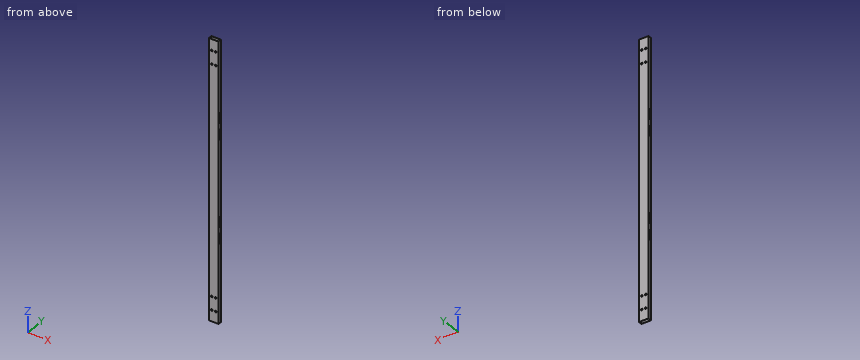
from build123d import *

# Parameters (mm, degrees)
SKETCH_1_W          = 40
SKETCH_1_H          = 15
SKETCH_1_W_2        = 38
SKETCH_1_H_2        = 13
EXTRUDE_1_DEPTH     = 1150
SKETCH_2_R          = 3.575
CUT_EXTRUDE_1_DEPTH = 1151.793204707
SKETCH_3_R          = 2.1
CUT_EXTRUDE_2_DEPTH = 1151.793204707


with BuildPart() as part:
    # 草图1 → 凸台-拉伸1 (new body)
    with BuildSketch(Plane.XY):
        with Locations((20, 7.5)):
            Rectangle(SKETCH_1_W, SKETCH_1_H)
        with Locations((20, 7.5)):
            Rectangle(SKETCH_1_W_2, SKETCH_1_H_2, mode=Mode.SUBTRACT)
    extrude(amount=EXTRUDE_1_DEPTH)

    # 草图2 → 切除-拉伸1 (cut, through all)
    with BuildSketch(Plane.XZ):
        with Locations(Location((12, 46, 0), (0, 0, 270))):
            Circle(SKETCH_2_R)
        with Locations(Location((28, 46, 0), (0, 0, 270))):
            Circle(SKETCH_2_R)
        with Locations(Location((12, 102, 0), (0, 0, 270))):
            Circle(SKETCH_2_R)
        with Locations(Location((28, 102, 0), (0, 0, 270))):
            Circle(SKETCH_2_R)
        with Locations(Location((12, 1104, 0), (0, 0, 270))):
            Circle(SKETCH_2_R)
        with Locations(Location((28, 1104, 0), (0, 0, 270))):
            Circle(SKETCH_2_R)
        with Locations(Location((12, 1048, 0), (0, 0, 270))):
            Circle(SKETCH_2_R)
        with Locations(Location((28, 1048, 0), (0, 0, 270))):
            Circle(SKETCH_2_R)
    extrude(amount=-CUT_EXTRUDE_1_DEPTH, mode=Mode.SUBTRACT)

    # 草图3 → 切除-拉伸2 (cut, through all)
    with BuildSketch(Plane(origin=(40, 0, 0), x_dir=(0, 0, -1), z_dir=(1, 0, 0))):
        with Locations((-430, 7)):
            Circle(SKETCH_3_R)
        with Locations((-418, 7)):
            Circle(SKETCH_3_R)
        with Locations((-338, 7)):
            Circle(SKETCH_3_R)
        with Locations((-326, 7)):
            Circle(SKETCH_3_R)
        with Locations((-406, 7)):
            Circle(SKETCH_3_R)
        with Locations((-394, 7)):
            Circle(SKETCH_3_R)
        with Locations((-362, 7)):
            Circle(SKETCH_3_R)
        with Locations((-350, 7)):
            Circle(SKETCH_3_R)
        with Locations((-854, 7)):
            Circle(SKETCH_3_R)
        with Locations((-842, 7)):
            Circle(SKETCH_3_R)
        with Locations((-762, 7)):
            Circle(SKETCH_3_R)
        with Locations((-750, 7)):
            Circle(SKETCH_3_R)
        with Locations((-830, 7)):
            Circle(SKETCH_3_R)
        with Locations((-818, 7)):
            Circle(SKETCH_3_R)
        with Locations((-786, 7)):
            Circle(SKETCH_3_R)
        with Locations((-774, 7)):
            Circle(SKETCH_3_R)
    extrude(amount=-CUT_EXTRUDE_2_DEPTH, mode=Mode.SUBTRACT)


solid = part.part
Here's how the part is built. I have some questions about the finished solid (model axes, mm). Give positions to 0.01 mm unless a question says otherwise; leave off trailing zeros. Order: outer loops, then holes, each group sorted by start corner. A loop starts at its lowest first (then second) coordinate and runs counter-clockwise, first axis right, second up. Notation, with made-up numbers: M 75.25,-22 L 98.25,-22 A20 ccw 98.25,-15 Z; hole C 61,-4 d9. An arc over 180 degrees is marked long. Answer as a JSON object with one key per item and string values. Group by question number.
1) Suppose I cut it at A-A, the plane z = 1023. Write out the boundary of the cut face in (x, y).
2) I'm going to push a flat-ended pin straight in: pin 1 Ø5.5 at (y, z) = (7, 350) entering from -X. Where does the tip first touch, or does it pass through?
3) Please list where these lines run through material, in increasing order: L1, parallel to X at y = 0.6, z = 46 (3 decimals); L2, parallel to X at y = 2.25, z = 744.5; L3, parallel to Y at x = 10.5, z = 409. Write a range as [from, to].
Results found:
{
 "1": {"outline": "M 0,0 L 40,0 L 40,15 L 0,15 Z; hole M 1,1 L 39,1 L 39,14 L 1,14 Z"},
 "2": {"pin 1": "x = 0"},
 "3": {"L1": "[0, 8.425], [15.575, 24.425], [31.575, 40]", "L2": "[0, 1], [39, 40]", "L3": "[0, 1], [14, 15]"}
}
